from build123d import *

# Parameters (mm, degrees)
EXTRUDE_1_DEPTH     = 15
SKETCH_7_W          = 10
SKETCH_7_H          = 12
SKETCH_7_W_2        = 4
SKETCH_7_H_2        = 4
CUT_EXTRUDE_1_DEPTH = 1
EXTRUDE_2_DEPTH     = 4.5
EXTRUDE_3_DEPTH     = 10
EXTRUDE_START       = 1
EXTRUDE_4_DEPTH     = 3.5


with BuildPart() as part:
    # 草图1 → 凸台-拉伸1 (new, symmetric)
    with BuildSketch(Plane.XY):
        Polygon((0, 0), (0, 40), (-8, 40), (-8, 2.886751346), (-3, 0), align=None)
    extrude(amount=EXTRUDE_1_DEPTH, both=True)

    # 草图7 → 切除-拉伸1 (cut)
    with BuildSketch(Plane.ZY.offset(8)):
        with Locations((0, 12)):
            Rectangle(SKETCH_7_W, SKETCH_7_H)
        with Locations((-10, 8)):
            Rectangle(SKETCH_7_W_2, SKETCH_7_H_2)
        with Locations((10, 8)):
            Rectangle(SKETCH_7_W_2, SKETCH_7_H_2)
    extrude(amount=-CUT_EXTRUDE_1_DEPTH, mode=Mode.SUBTRACT)

    # 草图9 → 凸台-拉伸2 (add, symmetric)
    with BuildSketch(Plane.XY):
        Polygon((-7, 14), (-8, 14), (-12, 13), (-12, 11), (-8, 10), (-7, 10), align=None)
    extrude(amount=EXTRUDE_2_DEPTH, both=True)

    # 草图15 → 凸台-拉伸3 (add, symmetric)
    with BuildSketch(Plane.XY):
        with BuildLine():
            Line((-8, 29), (-16, 29))
            ThreePointArc((-16, 29), (-18, 31), (-16, 33))
            Line((-16, 33), (-8, 33))
            ThreePointArc((-8, 33), (-6, 31), (-8, 29))
        make_face()
    extrude(amount=EXTRUDE_3_DEPTH, both=True)

    # 草图16 → 凸台-拉伸4 (add)
    with BuildSketch(Plane.XY.offset(15).offset(EXTRUDE_START)):
        with BuildLine():
            Line((-4, 18), (-12, 18))
            ThreePointArc((-12, 18), (-12.707106781, 18.292893219), (-13, 19))
            Line((-13, 19), (-13, 37))
            ThreePointArc((-13, 37), (-12.707106781, 37.707106781), (-12, 38))
            Line((-12, 38), (-4, 38))
            ThreePointArc((-4, 38), (-3.292893219, 37.707106781), (-3, 37))
            Line((-3, 37), (-3, 19))
            ThreePointArc((-3, 19), (-3.292893219, 18.292893219), (-4, 18))
        make_face()
    extrude_4 = extrude(amount=-EXTRUDE_4_DEPTH)

    # 镜向1: 凸台-拉伸4 across plane
    add(extrude_4.mirror(Plane.XY))


solid = part.part
Can you work these out from the model? Positions are in its coordinate system, mm. A direction names the side the tool comes from. Round coordinates to 2 decimals unless told otherwise and drop trailing zeros. Order: outer loops, then holes, each group sorted by start corner. A loop starts at its lowest first (then second) coordinate and runs counter-clockwise, first axis right, second up. Notation, with made-up numbers: M -7.5,72.5 L 30.5,72.5 A33 cw 30.5,108.5 Z; hole C -9.5,66 d5. An arc over 180 degrees is marked long. Use a Markdown table: item, result.
1) Imagine slicing it at A-A (x = -9.75). List the corners of the cut face in (y, z) for me, then the cut area to 3 significant figures.
Geometry says:
| item | result |
|---|---|
| outline | M 10.44,-4.5 L 13.56,-4.5 L 13.56,4.5 L 10.44,4.5 Z; M 18,-16 L 38,-16 L 38,-12.5 L 18,-12.5 Z; M 18,12.5 L 38,12.5 L 38,16 L 18,16 Z; M 29,-10 L 33,-10 L 33,10 L 29,10 Z |
| area | 248 mm² |
2) If we mould it in two halves opening along Y, with no side actions, what happens to faces 1 (the face through (-12.699, 18.285, -14.274)), 2 (the face through (-7.5, 6, 10)), 3 (the face through (-8, 28, -16))? For each: +Y half, -Y half, draft (parallel to the pull), parting line (faces both ways), or undercut.
Geometry says:
| item | result |
|---|---|
| face 1 | -Y half |
| face 2 | undercut |
| face 3 | draft |
3) Imagine slicing it at C-C (z = 5.5). List the corners of the cut face in (x, y) for me, then the cut area to 3 significant figures.
Geometry says:
| item | result |
|---|---|
| outline | M -16,29 L -8,29 L -8,2.89 L -3,0 L 0,0 L 0,40 L -8,40 L -8,33 L -16,33 A2 ccw Z |
| area | 351 mm² |
4) Imagine slicing it at B-B (y = 20.5). List the corners of the cut face in (x, z) for me, then the cut area to 3 significant figures.
Geometry says:
| item | result |
|---|---|
| outline | M -13,-16 L -3,-16 L -3,-15 L 0,-15 L 0,15 L -3,15 L -3,16 L -13,16 L -13,12.5 L -8,12.5 L -8,-12.5 L -13,-12.5 Z |
| area | 285 mm² |
5) Imagine slicing it at D-D (x = -15.5). List the corners of the cut face in (y, z) for me, then the cut area to 3 significant figures.
Geometry says:
| item | result |
|---|---|
| outline | M 29,-10 L 33,-10 L 33,10 L 29,10 Z |
| area | 80.0 mm² |
6) On a 3-axis mill with a long thin cutter (end or side, diameter ignored), from which of +Z, -Z, +X, -X, +Y, -Y can I reach the whole of each face in a straight line? I mean faces 4 (the face through (-10, 28, 12.5)), 5 (the face through (-3, 28.1, -15.5)), 6 (the face through (-7, 8, -10)). Say none if no direction works.
Geometry says:
| item | result |
|---|---|
| face 4 | -X, +Y, -Y |
| face 5 | -Z, +X, +Y, -Y |
| face 6 | -X |
7) I'm going to push flat-ended pins straight in: P1, Ø2, axis at x = -15, y = 32, coming from the -Z side; P2, Ø1.1, axis at x = -7.5, y = 8, coming from the +Z side; P3, Ø2.5, axis at x = -14, z = 0, coming from the +Y side. Where does each tip first touch, or does it pass through?
Geometry says:
| item | result |
|---|---|
| P1 | stops at z = -10 |
| P2 | stops at z = 15 |
| P3 | stops at y = 33 |
8) If I drill on line 1 along Z through (x, y) = (-12.25, 29.5); line 2 along Z through (x, y) = (-11.5, 28); line 3 along Y through (x, z) = (-13, 6.5), over which ranges is the centre line in solid material (lowest first)?
Geometry says:
| item | result |
|---|---|
| line 1 | z = -16 to -12.5, -10 to 10, 12.5 to 16 |
| line 2 | z = -16 to -12.5, 12.5 to 16 |
| line 3 | y = 29 to 33 |
